Autodesk Inventor part; units mm, degrees
ref_plane "YZ Plane" through (0, 0, 0) normal (1, 0, 0) x (0, 1, 0)
ref_plane "XZ Plane" through (0, 0, 0) normal (0, 1, 0) x (-1, 0, 0)
ref_plane "XY Plane" through (0, 0, 0) normal (0, 0, 1) x (1, 0, 0)
sketch "Szkic1" plane through (0, 0, 0) normal (0, 1, 0) x (-1, 0, 0)
  line L0 (0, 0) -> (0, -120)
  line L1 (0, -120) -> (0, 120)
  circle A0 centre (0, 120) radius 2
  circle A1 centre (0, -120) radius 2
  circle A2 centre (0, -120) radius 4
  circle A3 centre (0, 120) radius 4
  line L2 (-3, 117.3542) -> (3, 117.3542)
  line L3 (3, 117.3542) -> (3, -117.3542)
  line L4 (3, -117.3542) -> (-3, -117.3542)
  line L5 (-3, -117.3542) -> (-3, 117.3542)
  line L6 (3, 117.3542) -> (-3, 117.3542)
  line L7 (-3, 117.3542) -> (-3, 112.3542)
  line L8 (-3, 112.3542) -> (3, 112.3542)
  line L9 (3, 112.3542) -> (3, 117.3542)
  line L10 (3, -117.3542) -> (-3, -117.3542)
  line L11 (-3, -117.3542) -> (-3, -112.3542)
  line L12 (-3, -112.3542) -> (3, -112.3542)
  line L13 (3, -112.3542) -> (3, -117.3542)
  point P0 (-3, -117.3542)
  point P1 (3, -112.3542)
  point P2 (3, 112.3542)
  dimension "d4" = 8
  dimension "d5" = 8
  dimension "d0" = 120
  dimension "d1" = 240
  dimension "d2" = 4
  dimension "d3" = 4
  dimension "d6" = 3
  dimension "d7" = 3
  dimension "d14" = 5
  dimension "d15" = 5
extrude "Wyciągnięcie proste1" add sketch "Szkic1" along normal blind 3 contours L12 L3 A2 L0 | L0 A2 L5 L12 | L8 L5 A3 L1 | L1 A3 L3 L8 | A2 L4 L0 | L0 L4 A2 | A3 L2 L1 | L1 L2 A3 | L4 A2 | L2 A3
sketch "Szkic4" plane through (3, 0, 117.3542) normal (1, 0, 0) x (0, 0, -1)
  line L0 (0, 3) -> (5, 3)
  line L1 (2.5, 3) -> (232.2085, 3)
  line L2 (232.2085, 3) -> (117.3542, 3)
  line L3 (117.3542, 0) -> (117.3542, 27)
  line L4 (117.3542, 27) -> (177.3542, 27)
  line L5 (177.3542, 27) -> (57.3542, 27)
  arc A0 (57.3542, 27) -> (2.5, 3) centre (57.3542, -47.6873) ccw
  arc A1 (232.2085, 3) -> (177.3542, 27) centre (177.3542, -47.6873) ccw
  line L6 (57.3542, 27) -> (177.3542, 27)
  line L7 (177.3542, 27) -> (177.3542, 21)
  line L8 (177.3542, 21) -> (57.3542, 21)
  line L9 (57.3542, 21) -> (57.3542, 27)
  line L10 (0, 0) -> (5, 0)
  arc A2 (57.3542, 21) -> (5, 0) centre (57.3542, -54.7611) ccw
  line L11 (229.7085, 0) -> (229.7085, 3)
  arc A3 (229.7085, 0) -> (177.3542, 21) centre (177.3542, -54.7611) ccw
  line L12 (5, 0) -> (5, 3)
  point P0 (226.3787, 3)
  dimension "d26" = 27
  dimension "d27" = 60
  dimension "d28" = 120
  dimension "d29" = 6
extrude "Wyciągnięcie proste4" add sketch "Szkic4" against normal blind 6 contours A0 L9 A2 L1 L0 | L1 A2 L12 | L5 L3 L8 L9 | L4 L7 L8 L3 | A1 L1 A3 L7 | L1 L11 A3
properties part number "lacznik2"
Geometry: final body of the model. Coordinates: model frame, mm. A direction names the side the tool comes from. Give positions to 0.01 mm unless a question says otherwise; leave off trailing zeros. Write each loop counter-clockwise with the first axis right and the second up, starting at its lowest first coordinate (ties: lowest second). Pieces come first, ordered by that corner, then holes.
1. Reachability of faces 1 (the flat face through (0, 3, 117)), 2 (the cylindrical face through (0.042, 15.403, -88.58)), 3 (the flat face through (0, 3, -117)) from +Z, -Z, +X, -X, +Y, -Y: full face, straight path, thin tool, end or side. Return the list, or none.
2. Section query C-C, the plane y = 6.5. Return loops of the section in (x, z).
3. Draft query along Z for faces 4 (the cylindrical face through (0.042, 20.563, -90.332)), 5 (the cylindrical face through (0.04, 20.91, 89.54)), 6 (the cylindrical face through (0, 1, -124)), 7 (the flat face through (0, 27, -1)). Return one class per face: released by +Z, released by -Z, zero draft, split by the parting line, or undercut.
4. Section query A-A, the plane z = 120. Return loops of the section in (x, y), then the cut area to 3 significant figures.
5. Section query B-B, the plane x = 0. Count the separate pieces of the cut face and the enclosed holes in it, then the cut area to 3 significant figures.
6. Section query D-D, the plane z = -39. Return loops of the section in (x, y), then the cut area to 3 significant figures.
7. Line query: probe 1 along Z at (x, y) = (0, 0.8); probe 2 along Z at (x, y) = (0, 2.05); probe 3 along Y at (x, z) = (-1.5, -34). Output: solid intervals per line, ascending.
8. Pin query (flat end, axial travel): P1, Ø4, axis at y = 21.5, z = -51.5, coming from the +X side; P2, Ø4, axis at x = -1.5, z = -34, coming from the -Y side. Return the tip coordinate at first contact, or that it passes through.
Computed:
1. face 1: +Z, +X, -X, +Y
1. face 2: +X, -X, -Y
1. face 3: -Z, +X, -X, +Y
2. outline: (-3, -111.4) - (3, -111.4) - (3, -104.57) - (-3, -104.57) - close; (-3, 104.57) - (3, 104.57) - (3, 111.4) - (-3, 111.4) - close
3. face 4: released by -Z
3. face 5: released by +Z
3. face 6: undercut
3. face 7: zero draft
4. outline: (-4, 0) - (-2, 0) - (-2, 3) - (-4, 3) - close; (2, 0) - (4, 0) - (4, 3) - (2, 3) - close
4. area: 12.0 mm2
5. separate pieces: 3
5. enclosed holes: 0
5. area: 1,390 mm2
6. outline: (-3, 21) - (3, 21) - (3, 27) - (-3, 27) - close
6. area: 36.0 mm2
7. probe 1: z = -124 to -122, -118 to -111.5, 111.5 to 118, 122 to 124
7. probe 2: z = -124 to -122, -118 to -110.12, 110.12 to 118, 122 to 124
7. probe 3: y = 21 to 27
8. P1: stops at x = 3
8. P2: stops at y = 21
